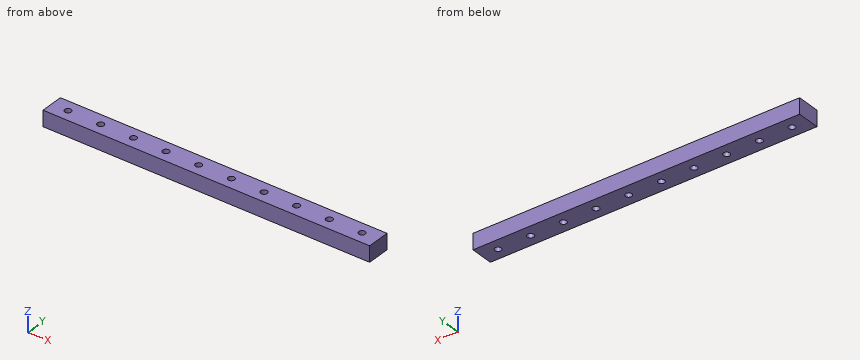
```python
from build123d import *

# Parameters (mm, degrees)
SKETCH_1_W          = 100
SKETCH_1_H          = 7
EXTRUDE_1_DEPTH     = 4.8
SKETCH_2_R          = 1
CUT_EXTRUDE_1_DEPTH = 4.8


with BuildPart() as part:
    # 草图1 → 凸台-拉伸1 (new body)
    with BuildSketch(Plane.XY):
        with Locations((50, 3.5)):
            Rectangle(SKETCH_1_W, SKETCH_1_H)
    extrude(amount=EXTRUDE_1_DEPTH)

    # 草图2 → 切除-拉伸1 (cut)
    with BuildSketch(Plane.XY.offset(4.8)):
        with BuildLine():
            ThreePointArc((6, 3.5), (5, 4.5), (4, 3.5))
            Line((4, 3.5), (6, 3.5))
        make_face()
        with BuildLine():
            Line((6, 3.5), (4, 3.5))
            ThreePointArc((4, 3.5), (5, 2.5), (6, 3.5))
        make_face()
        with BuildLine():
            ThreePointArc((16, 3.5), (15, 4.5), (14, 3.5))
            Line((14, 3.5), (16, 3.5))
        make_face()
        with BuildLine():
            Line((16, 3.5), (14, 3.5))
            ThreePointArc((14, 3.5), (15, 2.5), (16, 3.5))
        make_face()
        with BuildLine():
            ThreePointArc((26, 3.5), (25, 4.5), (24, 3.5))
            Line((24, 3.5), (26, 3.5))
        make_face()
        with BuildLine():
            Line((26, 3.5), (24, 3.5))
            ThreePointArc((24, 3.5), (25, 2.5), (26, 3.5))
        make_face()
        with BuildLine():
            ThreePointArc((36, 3.5), (35, 4.5), (34, 3.5))
            Line((34, 3.5), (36, 3.5))
        make_face()
        with BuildLine():
            Line((36, 3.5), (34, 3.5))
            ThreePointArc((34, 3.5), (35, 2.5), (36, 3.5))
        make_face()
        with BuildLine():
            ThreePointArc((46, 3.5), (45, 4.5), (44, 3.5))
            Line((44, 3.5), (46, 3.5))
        make_face()
        with BuildLine():
            Line((46, 3.5), (44, 3.5))
            ThreePointArc((44, 3.5), (45, 2.5), (46, 3.5))
        make_face()
        with BuildLine():
            ThreePointArc((56, 3.5), (55, 4.5), (54, 3.5))
            Line((54, 3.5), (56, 3.5))
        make_face()
        with BuildLine():
            Line((56, 3.5), (54, 3.5))
            ThreePointArc((54, 3.5), (55, 2.5), (56, 3.5))
        make_face()
        with BuildLine():
            ThreePointArc((76, 3.5), (75, 4.5), (74, 3.5))
            Line((74, 3.5), (76, 3.5))
        make_face()
        with BuildLine():
            Line((76, 3.5), (74, 3.5))
            ThreePointArc((74, 3.5), (75, 2.5), (76, 3.5))
        make_face()
        with BuildLine():
            ThreePointArc((86, 3.5), (85, 4.5), (84, 3.5))
            Line((84, 3.5), (86, 3.5))
        make_face()
        with BuildLine():
            Line((86, 3.5), (84, 3.5))
            ThreePointArc((84, 3.5), (85, 2.5), (86, 3.5))
        make_face()
        with BuildLine():
            ThreePointArc((96, 3.5), (95, 4.5), (94, 3.5))
            Line((94, 3.5), (96, 3.5))
        make_face()
        with BuildLine():
            Line((96, 3.5), (94, 3.5))
            ThreePointArc((94, 3.5), (95, 2.5), (96, 3.5))
        make_face()
        with Locations((65, 3.5)):
            Circle(SKETCH_2_R)
    extrude(amount=-CUT_EXTRUDE_1_DEPTH, mode=Mode.SUBTRACT)


solid = part.part
```
Here's how the part is built. I have some questions about the finished solid (model axes, mm). Coordinates: 2 decimals unless noted, no trailing zeros. Loops run counter-clockwise (first coordinate to the right, second up) from the corner with the lowest first, then second, coordinate; pieces in that order, holes last. Notation, with made-up numbers: (25.5, 20) -> (46.5, 20) arc R34 cw to (46.5, 50) -> close; hole circle Ø7 at (52, 88). An arc over 180 degrees is marked (long way). Return JSON: item names as keys, results as strings.
1) If we section it at B-B, the plane z = 3.25: Count the separate pieces of the cut face and the enclosed holes in it, then the cut area to 3 significant figures.
Results below:
{"separate pieces": "1", "enclosed holes": "10", "area": "669 mm²"}
2) I need wall thicknesses on line 1 (Y direction, x = 15, z = 1.7). Which ranges of the line are inside material? Lowest first, please. Write a range as from..to.
Results below:
{"line 1": "0..2.5, 4.5..7"}
3) If we section it at A-A, the plane x = 15: Write out the boundary of the cut face in (y, z).
Results below:
{"outline": "(0, 0) -> (2.5, 0) -> (2.5, 4.8) -> (0, 4.8) -> close; (4.5, 0) -> (7, 0) -> (7, 4.8) -> (4.5, 4.8) -> close"}
